Answer from the drawing. Dimensions are ordinates in mm from the lowest x, y and z of the part. A direction names the side the tool comes from. Give positions to 0.01 mm unless a question says otherwise; leave off trailing zeros. Order: outer loops, then holes, each group sorted by start corner. A loop starts at its lowest first (then second) coordinate and runs counter-clockwise, first axis right, second up. Notation, with made-up numbers: (59, -10.5) - (113, -10.5) arc R28 ccw to (113, 9.5) - close; hole circle Ø9 at (-24, 82). An arc over 180 degrees is marked (long way). Write each question's results on one line, items separated by ' | '.
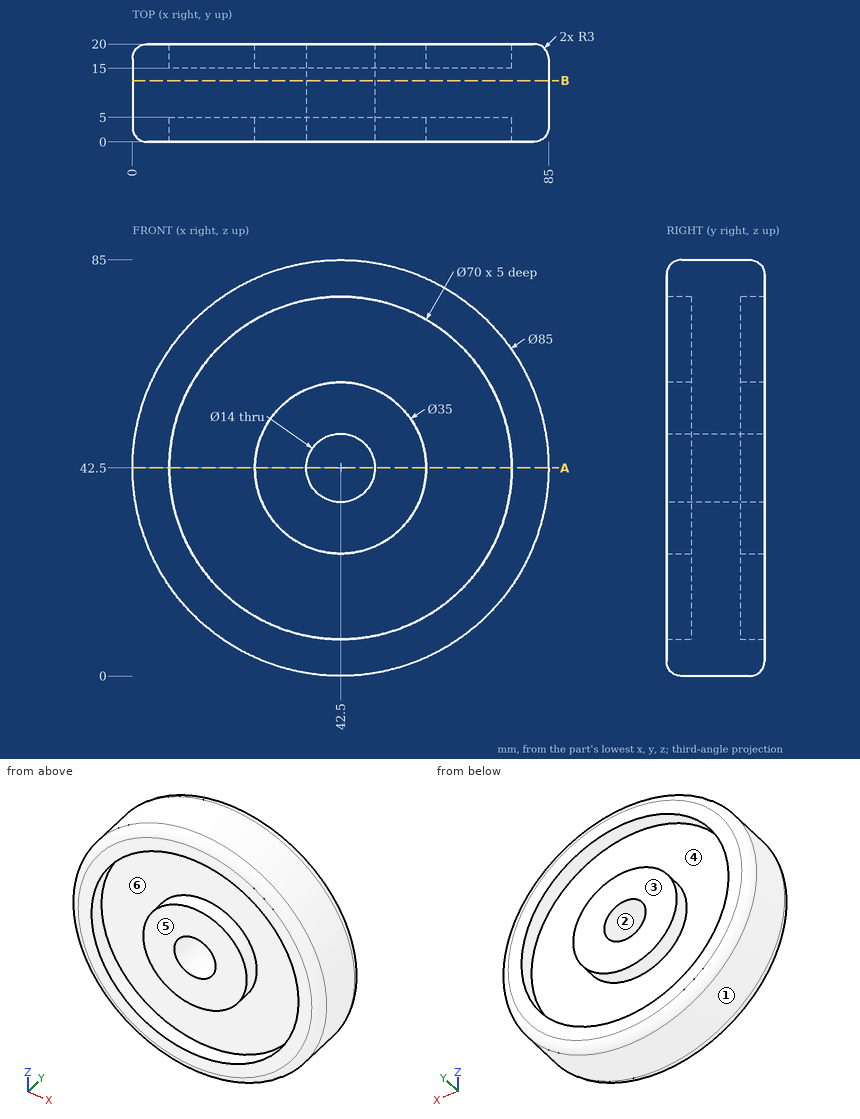
1. A cutting plane is placed at A-A, the plane z = 42.5. Write down the section's boundary in (x, y), then the cut area to 3 significant figures.
Answer list:
outline: (0, 3) arc R3 ccw to (3, 0) - (7.5, 0) - (7.5, 5) - (25, 5) - (25, 0) - (35.5, 0) - (35.5, 20) - (25, 20) - (25, 15) - (7.5, 15) - (7.5, 20) - (3, 20) arc R3 ccw to (0, 17) - close; (49.5, 0) - (60, 0) - (60, 5) - (77.5, 5) - (77.5, 0) - (82, 0) arc R3 ccw to (85, 3) - (85, 17) arc R3 ccw to (82, 20) - (77.5, 20) - (77.5, 15) - (60, 15) - (60, 20) - (49.5, 20) - close | area: 1,060 mm^2
2. A tool of negligible diameter and unlimited length cuts with its end or side. For the marked faces 5 and 6, from which of +Z, -Z, +X, -X, +Y, -Y can it reach the whole face along a straight path? Write none if from no direction.
Answer list:
face 5: +Z, -Z, +X, -X, -Y | face 6: -Y
3. Straight lines are drawn through the part: line 1 (X direction, y = 3.2, z = 42.5); line 2 (Z direction, x = 39.5, y = 4.5); line 3 (X direction, y = 1.2, z = 42.5). For each, find the intervals that lie inside material, in ascending order. Write a range as [from, to].
Answer list:
line 1: [0, 7.5], [25, 35.5], [49.5, 60], [77.5, 85] | line 2: [0.11, 7.63], [25.26, 36.18], [48.82, 59.74], [77.37, 84.89] | line 3: [0.6, 7.5], [25, 35.5], [49.5, 60], [77.5, 84.4]
4. Given P1, Ø5, axis at y = 6.5, z = 75.5, coming from the -X side; P2, Ø4, axis at x = 71, y = 18, coming from the +Z side; P3, Ø5, axis at y = 6, z = 57.5, coming from the +X side; P4, Ø12, axis at x = 72, z = 13, coming from the +Y side, each flat-ended and moving along its own axis, determine where each tip first touches the part or whether it passes through.
Answer list:
P1: x = 12.9 | P2: z = 75.62 | P3: x = 83.12 | P4: y = 20
5. A cutting plane is placed at B-B, the plane y = 12.5. Write down the section's boundary in (x, z).
Answer list:
outline: circle Ø85 at (42.5, 42.5); hole circle Ø14 at (42.5, 42.5)
6. Determine the mould class of the marked faces 1, 2, 3 and 4 for opening direction X: +X half, -X half, draft (parallel to the pull), parting line (faces both ways), or undercut.
Answer list:
face 1: parting line | face 2: undercut | face 3: draft | face 4: undercut
